The model under review builds one solid part; all positions refer to its coordinate system, in mm. A direction names the side the tool comes from. Give positions to 0.01 mm unless a question says otherwise; leave off trailing zeros. Loops run counter-clockwise (first coordinate to the right, second up) from the corner with the lowest first, then second, coordinate; pieces in that order, holes last. Notation, with made-up numbers: M 47,86.25 L 72,86.25 A19 cw 72,114.25 Z; hole C 55,14 d3. An arc over 180 degrees is marked long. Return JSON: item names as keys, results as strings.
```python
from build123d import *

# Parameters (mm, degrees)
SZKIC2_R                   = 3
WYTNIJ_WYCI_GNI_CIE1_DEPTH = 13


with BuildPart() as part:
    # Szkic1 → Obrót5 (revolve)
    with BuildSketch(Plane.XY, mode=Mode.PRIVATE) as obr_t5_sk:
        with BuildLine():
            Line((-10, 0), (-5, 0))
            Line((-5, 0), (-5, 8))
            Line((-5, 8), (-6, 8))
            Line((-6, 8), (-6, 13))
            Line((-6, 13), (0, 13))
            Line((0, 13), (0, 0))
            Line((0, 0), (0, -10))
            ThreePointArc((0, -10), (-7.071067812, -7.071067812), (-10, 0))
        make_face()
    revolve(obr_t5_sk.sketch.rotate(Axis((0, -10, 0), (0, 1, 0)), 180), axis=Axis((0, -10, 0), (0, 1, 0)))

    # Szkic2 → Wytnij-wyciągnięcie1 (cut)
    with BuildSketch(Plane(origin=(0, 13, 0), x_dir=(1, 0, 0), z_dir=(0, 1, 0))):
        with Locations(Location((0, 0, 0), (0, 0, 180))):
            Circle(SZKIC2_R)
    extrude(amount=-WYTNIJ_WYCI_GNI_CIE1_DEPTH, mode=Mode.SUBTRACT)


solid = part.part
```
1) The part is to be moulded in two halves that separate along Y. For faces 3 (the face through (4, 8, -4)), 4 (the face through (-2.86, 6.59, 0.9)), 5 (the face through (0, 0, 0)), 6 (the face through (-5, 4, 0)), say which applies: released by +Y, released by -Y, zero draft, split by the parting line, or undercut.
From the geometry:
{"face 3": "undercut", "face 4": "zero draft", "face 5": "released by +Y", "face 6": "undercut"}
2) Consider section A-A on z = 0. Write out the cut boundary in (x, y), then the cut area to 3 significant figures.
From the geometry:
{"outline": "M -10,0 A10 ccw 10,0 L 5,0 L 5,8 L 6,8 L 6,13 L 3,13 L 3,0 L -3,0 L -3,13 L -6,13 L -6,8 L -5,8 L -5,0 Z", "area": "219 mm²"}
3) Wall thickness on L1, parallel to Z at x = 0, y = 5.5; L2, parallel to Z at x = 0, y = 8.5; L3, parallel to X at y = 1.25, z = -2.5: over which ranges is each line inside the solid? List them lowest first. Write a range as from..to.
From the geometry:
{"L1": "-5..-3, 3..5", "L2": "-6..-3, 3..6", "L3": "-4.33..-1.66, 1.66..4.33"}
4) Tool access review of faces 1 (the face through (-3, 13, 1)), 2 (the face through (5.723, 10.535, -1.802)): name each direction out of +Z, -Z, +X, -X, +Y, -Y from which nothing blocks a thin tool from reaching the whole face with its end or side.
From the geometry:
{"face 1": "+Z, -Z, +X, -X, +Y", "face 2": "+Y"}
5) Insertion check: pin 1 (9.5 mm diameter, centred on x = 0, z = 1, fed in from -Y); pin 2 (10 mm diameter, centred on x = 4.5, y = -7.5, fed in from +Z); pin 3 (1.8 mm diameter, centred on x = 0.5, z = -1, fed in from +Y); pin 4 (5 mm diameter, centred on x = 7.5, y = -2, fed in from +Z). Each pin has a flat end and moves straight along its axis. Give the tip position at first contact, or say it passes through.
From the geometry:
{"pin 1": "y = -10", "pin 2": "z = 9.27", "pin 3": "y = 0", "pin 4": "z = 8.5"}
6) Consider section C-C on y = 4.5. Write out the cut boundary in (x, z), then the cut area to 3 significant figures.
From the geometry:
{"outline": "C 0,0 d10; hole C 0,0 d6", "area": "50.3 mm²"}
7) Consider section D-D on x = 3.5. Write out the cut boundary in (y, z) (1 decimal).
From the geometry:
{"outline": "M 0,-9.4 L 0,-3.6 L 8,-3.6 L 8,-4.9 L 13,-4.9 L 13,4.9 L 8,4.9 L 8,3.6 L 0,3.6 L 0,9.4 A9.4 ccw Z"}
8) Consider section B-B on x = 0. Write out the cut boundary in (y, z), then the cut area to 3 significant figures.
From the geometry:
{"outline": "M 0,-10 L 0,-5 L 8,-5 L 8,-6 L 13,-6 L 13,-3 L 0,-3 L 0,3 L 13,3 L 13,6 L 8,6 L 8,5 L 0,5 L 0,10 A10 ccw Z", "area": "219 mm²"}
